```python
from build123d import *

# Parameters (mm, degrees)
F0_R     = 2.6035
F1_DEPTH = 25.4


with BuildPart() as f1:
    # F0 (on Front) → F1 (new body)
    with BuildSketch(Plane.XZ):
        with BuildLine():
            Line((-17.0434, 12.828983), (-23.2918, 12.828983))
            ThreePointArc((-23.2918, 12.828983), (-24.782523, 12.211505), (-25.4, 10.720783))
            Line((-25.4, 10.720783), (-25.4, 4.472383))
            ThreePointArc((-25.4, 4.472383), (-24.2951, 3.367483), (-23.1902, 4.472383))
            Line((-23.1902, 4.472383), (-23.1902, 6.528513))
            ThreePointArc((-23.1902, 6.528513), (-22.55203, 7.483601), (-21.425427, 7.259505))
            Line((-21.425427, 7.259505), (-18.138436, 3.972514))
            ThreePointArc((-18.138436, 3.972514), (-17.450182, 2.94247), (-17.2085, 1.72745))
            Line((-17.2085, 1.72745), (-17.2085, -1.469485))
            ThreePointArc((-17.2085, -1.469485), (-17.450182, -2.684505), (-18.138436, -3.714549))
            Line((-18.138436, -3.714549), (-21.425427, -7.00154))
            ThreePointArc((-21.425427, -7.00154), (-22.55203, -7.225636), (-23.1902, -6.270547))
            Line((-23.1902, -6.270547), (-23.1902, -4.214417))
            ThreePointArc((-23.1902, -4.214417), (-24.2951, -3.109517), (-25.4, -4.214417))
            Line((-25.4, -4.214417), (-25.4, -10.462817))
            ThreePointArc((-25.4, -10.462817), (-24.782523, -11.95354), (-23.2918, -12.571017))
            Line((-23.2918, -12.571017), (-17.0434, -12.571017))
            ThreePointArc((-17.0434, -12.571017), (-15.9385, -11.466117), (-17.0434, -10.361217))
            Line((-17.0434, -10.361217), (-19.09953, -10.361217))
            ThreePointArc((-19.09953, -10.361217), (-20.054618, -9.723048), (-19.830523, -8.596445))
            Line((-19.830523, -8.596445), (-16.543532, -5.309453))
            ThreePointArc((-16.543532, -5.309453), (-15.513488, -4.6212), (-14.298468, -4.379517))
            Line((-14.298468, -4.379517), (-11.101532, -4.379517))
            ThreePointArc((-11.101532, -4.379517), (-9.886512, -4.6212), (-8.856468, -5.309453))
            Line((-8.856468, -5.309453), (-5.569477, -8.596445))
            ThreePointArc((-5.569477, -8.596445), (-5.345382, -9.723048), (-6.30047, -10.361217))
            Line((-6.30047, -10.361217), (-8.3566, -10.361217))
            ThreePointArc((-8.3566, -10.361217), (-9.4615, -11.466117), (-8.3566, -12.571017))
            Line((-8.3566, -12.571017), (2.1082, -12.571017))
            Line((2.1082, -12.571017), (8.3566, -12.571017))
            ThreePointArc((8.3566, -12.571017), (9.4615, -11.466117), (8.3566, -10.361217))
            Line((8.3566, -10.361217), (6.30047, -10.361217))
            ThreePointArc((6.30047, -10.361217), (5.345382, -9.723048), (5.569477, -8.596445))
            Line((5.569477, -8.596445), (8.856468, -5.309453))
            ThreePointArc((8.856468, -5.309453), (9.886512, -4.6212), (11.101532, -4.379517))
            Line((11.101532, -4.379517), (14.298468, -4.379517))
            ThreePointArc((14.298468, -4.379517), (15.513488, -4.6212), (16.543532, -5.309453))
            Line((16.543532, -5.309453), (19.830523, -8.596445))
            ThreePointArc((19.830523, -8.596445), (20.054618, -9.723048), (19.09953, -10.361217))
            Line((19.09953, -10.361217), (17.0434, -10.361217))
            ThreePointArc((17.0434, -10.361217), (15.9385, -11.466117), (17.0434, -12.571017))
            Line((17.0434, -12.571017), (23.2918, -12.571017))
            ThreePointArc((23.2918, -12.571017), (24.782523, -11.95354), (25.4, -10.462817))
            Line((25.4, -10.462817), (25.4, -4.214417))
            ThreePointArc((25.4, -4.214417), (24.2951, -3.109517), (23.1902, -4.214417))
            Line((23.1902, -4.214417), (23.1902, -6.270547))
            ThreePointArc((23.1902, -6.270547), (22.55203, -7.225636), (21.425427, -7.00154))
            Line((21.425427, -7.00154), (18.138436, -3.714549))
            ThreePointArc((18.138436, -3.714549), (17.450182, -2.684505), (17.2085, -1.469485))
            Line((17.2085, -1.469485), (17.2085, 1.72745))
            ThreePointArc((17.2085, 1.72745), (17.450182, 2.94247), (18.138436, 3.972514))
            Line((18.138436, 3.972514), (21.425427, 7.259505))
            ThreePointArc((21.425427, 7.259505), (22.55203, 7.483601), (23.1902, 6.528513))
            Line((23.1902, 6.528513), (23.1902, 4.472383))
            ThreePointArc((23.1902, 4.472383), (24.2951, 3.367483), (25.4, 4.472383))
            Line((25.4, 4.472383), (25.4, 10.720783))
            ThreePointArc((25.4, 10.720783), (24.782523, 12.211505), (23.2918, 12.828983))
            Line((23.2918, 12.828983), (17.0434, 12.828983))
            ThreePointArc((17.0434, 12.828983), (15.9385, 11.724083), (17.0434, 10.619183))
            Line((17.0434, 10.619183), (19.09953, 10.619183))
            ThreePointArc((19.09953, 10.619183), (20.054618, 9.981013), (19.830523, 8.85441))
            Line((19.830523, 8.85441), (16.543532, 5.567419))
            ThreePointArc((16.543532, 5.567419), (15.513488, 4.879165), (14.298468, 4.637483))
            Line((14.298468, 4.637483), (11.101532, 4.637483))
            ThreePointArc((11.101532, 4.637483), (9.886512, 4.879165), (8.856468, 5.567419))
            Line((8.856468, 5.567419), (5.569477, 8.85441))
            ThreePointArc((5.569477, 8.85441), (5.345382, 9.981013), (6.30047, 10.619183))
            Line((6.30047, 10.619183), (8.3566, 10.619183))
            ThreePointArc((8.3566, 10.619183), (9.4615, 11.724083), (8.3566, 12.828983))
            Line((8.3566, 12.828983), (2.1082, 12.828983))
            Line((2.1082, 12.828983), (-8.3566, 12.828983))
            ThreePointArc((-8.3566, 12.828983), (-9.4615, 11.724083), (-8.3566, 10.619183))
            Line((-8.3566, 10.619183), (-6.30047, 10.619183))
            ThreePointArc((-6.30047, 10.619183), (-5.345382, 9.981013), (-5.569477, 8.85441))
            Line((-5.569477, 8.85441), (-8.856468, 5.567419))
            ThreePointArc((-8.856468, 5.567419), (-9.886512, 4.879165), (-11.101532, 4.637483))
            Line((-11.101532, 4.637483), (-14.298468, 4.637483))
            ThreePointArc((-14.298468, 4.637483), (-15.513488, 4.879165), (-16.543532, 5.567419))
            Line((-16.543532, 5.567419), (-19.830523, 8.85441))
            ThreePointArc((-19.830523, 8.85441), (-20.054618, 9.981013), (-19.09953, 10.619183))
            Line((-19.09953, 10.619183), (-17.0434, 10.619183))
            ThreePointArc((-17.0434, 10.619183), (-15.9385, 11.724083), (-17.0434, 12.828983))
        make_face()
        with Locations((-12.7, 0.128983)):
            Circle(F0_R, mode=Mode.SUBTRACT)
        with Locations((12.7, 0.128983)):
            Circle(F0_R, mode=Mode.SUBTRACT)
    extrude(amount=F1_DEPTH)


solid = f1.part
```
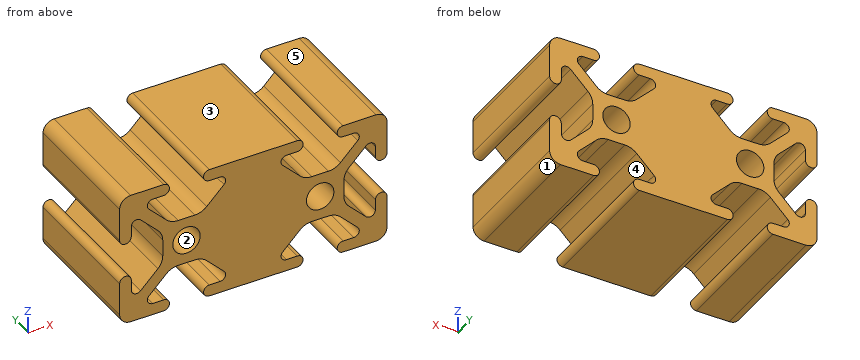
Can you work these out from the model? Positions are in its coordinate system, mm. Face numbers are marked on the shaded views. A direction names the side the tool comes from. Coordinates: 2 decimals unless noted, no trailing zeros. Order: outer loops, then holes, each group sorted by start corner. A loop starts at its lowest first (then second) coordinate and runs counter-clockwise, first axis right, second up.
1. Thinking about a two-plate mould opening in Z: for the marked faces 1, 2 and 3, which applies, +Z half, -Z half, draft (parallel to the pull), parting line (faces both ways), or undercut?
2. If we section it at A-A (x = -12.7): Please give me the cut outline in (y, z).
3. I need wall thicknesses on line 1 (Z direction, x = -12.7, y = -18); line 2 (X direction, y = -20.5, z = 10.5); line 3 (Z direction, x = 19, y = -5). Which ranges of each line are inside material? Lowest first, please.
4. If we section it at C-C (y = -14.25): Give the number of separate pieces and of enclosed holes in the cut face, then the cut area to 3 significant figures.
5. I'm going to push flat-ended pins straight in: pin 1 (2 mm diameter, centred on y = -18.5, z = -4, fed in from +X); pin 2 (3.5 mm diameter, centred on x = 12, y = -10.5, fed in from +Z); pin 3 (1 mm diameter, centred on x = -9, y = -15.5, fed in from +Z); pin 4 (2.5 mm diameter, centred on x = 12.5, y = -17.5, fed in from -Z). Where does each tip first touch, or does it pass through?
6. If we section it at B-B (z = 10): Please give me the cut outline in (x, y).
7. For the marked faces 4 and 5, which set-ups out of +Z, -Z, +X, -X, +Y, -Y let a thin tool reach every point of the face, with its end or its side?
Entries:
1. face 1: -Z half
1. face 2: undercut
1. face 3: +Z half
2. outline: (-25.4, -4.38) - (0, -4.38) - (0, -2.47) - (-25.4, -2.47) - close; (-25.4, 2.73) - (0, 2.73) - (0, 4.64) - (-25.4, 4.64) - close
3. line 1: z = -4.38 to -2.47, 2.73 to 4.64
3. line 2: x = -25.4 to -19.58, -5.82 to 5.82, 19.58 to 25.4
3. line 3: z = -12.57 to -10.36, -7.77 to -4.58, 4.83 to 8.02, 10.62 to 12.83
4. separate pieces: 1
4. enclosed holes: 2
4. area: 746 mm2
5. pin 1: stops at x = 25.4
5. pin 2: stops at z = 4.75
5. pin 3: stops at z = 12.82
5. pin 4: stops at z = -4.38
6. outline: (-25.4, -25.4) - (-20.05, -25.4) - (-20.05, 0) - (-25.4, 0) - close; (-5.35, -25.4) - (5.35, -25.4) - (5.35, 0) - (-5.35, 0) - close; (20.05, -25.4) - (25.4, -25.4) - (25.4, 0) - (20.05, 0) - close
7. face 4: +Y, -Y
7. face 5: +Z, +X, -X, +Y, -Y
